Source: CAD feature listing. Evaluate the final solid. Frame: model axes, mm. Face numbers are marked on the shaded views. A direction names the side the tool comes from. Round coordinates to 2 decimals unless told otherwise and drop trailing zeros. Loops run counter-clockwise (first coordinate to the right, second up) from the corner with the lowest first, then second, coordinate; pieces in that order, holes last. Notation, with made-up numbers: (-21, 30) - (-2, 30) arc R22 ccw to (-2, 38) - close; hole circle Ø2 at (-28.5, -8). An arc over 180 degrees is marked (long way). One line per question, with ' | ' between items.
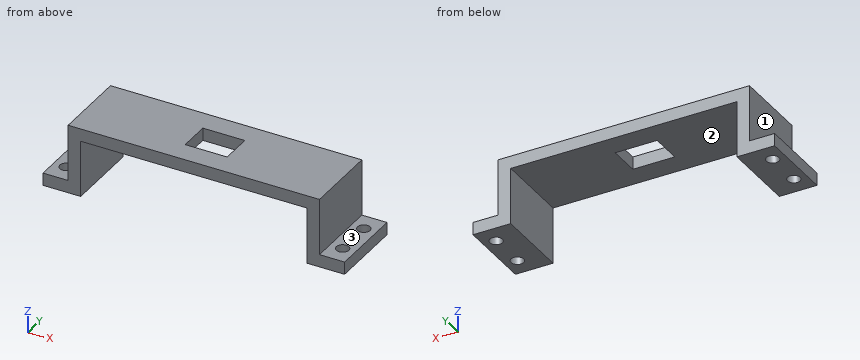
from build123d import *

# Parameters (mm, degrees)
SKETCH1_W           = 127
SKETCH1_H           = 38.1
SKETCH1_W_2         = 21.209
SKETCH1_H_2         = 15.88008
BOSS_EXTRUDE1_DEPTH = 6.35
SKETCH2_W           = 6.35
SKETCH2_H           = 38.1
BOSS_EXTRUDE2_DEPTH = 28.575
SKETCH3_W           = 6.35
SKETCH3_H           = 38.1
BOSS_EXTRUDE3_DEPTH = 12.7
SKETCH4_W           = 6.35
SKETCH4_H           = 38.1
BOSS_EXTRUDE4_DEPTH = 12.7
CUT_EXTRUDE1_REACH  = 149.595
SKETCH5_R           = 3.175


with BuildPart() as part:
    # Sketch1 → Boss-Extrude1 (new body)
    with BuildSketch(Plane.XY):
        with Locations((63.5, 19.05)):
            Rectangle(SKETCH1_W, SKETCH1_H)
        with Locations((63.5, 19.05)):
            Rectangle(SKETCH1_W_2, SKETCH1_H_2, mode=Mode.SUBTRACT)
    extrude(amount=BOSS_EXTRUDE1_DEPTH)

    # Sketch2 → Boss-Extrude2 (add)
    with BuildSketch(Plane(origin=(0, 0, 0), x_dir=(-1, 0, 0), z_dir=(0, 0, -1))):
        with Locations((-3.175, 19.05)):
            Rectangle(SKETCH2_W, SKETCH2_H)
        with Locations((-123.825, 19.05)):
            Rectangle(SKETCH2_W, SKETCH2_H)
    extrude(amount=BOSS_EXTRUDE2_DEPTH)

    # Sketch3 → Boss-Extrude3 (add)
    with BuildSketch(Plane(origin=(127, 0, 0), x_dir=(0, 0, -1), z_dir=(1, 0, 0))):
        with Locations((25.4, 19.05)):
            Rectangle(SKETCH3_W, SKETCH3_H)
    extrude(amount=BOSS_EXTRUDE3_DEPTH)

    # Sketch4 → Boss-Extrude4 (add)
    with BuildSketch(Plane.ZY):
        with Locations((-25.4, 19.05)):
            Rectangle(SKETCH4_W, SKETCH4_H)
    extrude(amount=BOSS_EXTRUDE4_DEPTH)

    # Sketch5 → Cut-Extrude1 (cut, up to next)
    with BuildSketch(Plane.XY.offset(-22.225), mode=Mode.PRIVATE) as cut_extrude1_sk1:
        with Locations((133.35, 28.575)):
            Circle(SKETCH5_R)
    cut_extrude1_tool1 = extrude(cut_extrude1_sk1.sketch, amount=-CUT_EXTRUDE1_REACH, mode=Mode.PRIVATE) & part.part
    # Sketch5 → Cut-Extrude1 (cut, up to next)
    with BuildSketch(Plane.XY.offset(-22.225), mode=Mode.PRIVATE) as cut_extrude1_sk2:
        with Locations((133.35, 9.525)):
            Circle(SKETCH5_R)
    cut_extrude1_tool2 = extrude(cut_extrude1_sk2.sketch, amount=-CUT_EXTRUDE1_REACH, mode=Mode.PRIVATE) & part.part
    # Sketch5 → Cut-Extrude1 (cut, up to next)
    with BuildSketch(Plane.XY.offset(-22.225), mode=Mode.PRIVATE) as cut_extrude1_sk3:
        with Locations((-6.35, 28.575)):
            Circle(SKETCH5_R)
    cut_extrude1_tool3 = extrude(cut_extrude1_sk3.sketch, amount=-CUT_EXTRUDE1_REACH, mode=Mode.PRIVATE) & part.part
    # Sketch5 → Cut-Extrude1 (cut, up to next)
    with BuildSketch(Plane.XY.offset(-22.225), mode=Mode.PRIVATE) as cut_extrude1_sk4:
        with Locations((-6.35, 9.525)):
            Circle(SKETCH5_R)
    cut_extrude1_tool4 = extrude(cut_extrude1_sk4.sketch, amount=-CUT_EXTRUDE1_REACH, mode=Mode.PRIVATE) & part.part
    add(cut_extrude1_tool1.solids().sort_by_distance((133.35, 28.575, -22.225))[0], mode=Mode.SUBTRACT)
    add(cut_extrude1_tool2.solids().sort_by_distance((133.35, 9.525, -22.225))[0], mode=Mode.SUBTRACT)
    add(cut_extrude1_tool3.solids().sort_by_distance((-6.35, 28.575, -22.225))[0], mode=Mode.SUBTRACT)
    add(cut_extrude1_tool4.solids().sort_by_distance((-6.35, 9.525, -22.225))[0], mode=Mode.SUBTRACT)


solid = part.part
1. Section query A-A, the plane x = -6.35. Return loops of the section in (y, z) (3 decimals).
Worked out:
outline: (0, -28.575) - (6.35, -28.575) - (6.35, -22.225) - (0, -22.225) - close; (12.7, -28.575) - (25.4, -28.575) - (25.4, -22.225) - (12.7, -22.225) - close; (31.75, -28.575) - (38.1, -28.575) - (38.1, -22.225) - (31.75, -22.225) - close
2. Access query for the marked faces 1, 2 and 3. Directions: +Z, -Z, +X, -X, +Y, -Y. A direction counts if a zero-diameter tool reaches every point of the face in a straight line with its end or side. Return the directions, or none.
Worked out:
face 1: +Z, -X, +Y, -Y | face 2: -Z, +Y, -Y | face 3: +Z, +X, +Y, -Y
3. Contact query for flat-ended pins moving along their axis: P1, Ø1.9, axis at y = 17.5, z = 3, coming from the -X side; P2, Ø5, axis at x = 133.35, y = 28.575, coming from the -Z side; P3, Ø1.9, axis at y = 21, z = 3.5, coming from the +X side; P4, Ø4, axis at x = 131, y = 13, coming from the +Z side (3 decimals). Output: stop coordinate, or through.
Worked out:
P1: stops at x = 0 | P2: passes through | P3: stops at x = 127 | P4: stops at z = -22.225
4. Material intervals for probe 1 along Y at (x, z) = (133, -24); probe 2 along X at (y, z) = (14.5, -14); probe 3 along X at (y, z) = (13, 4), sorted ascending.
Worked out:
probe 1: y = 0 to 6.37, 12.68 to 25.42, 31.73 to 38.1 | probe 2: x = 0 to 6.35, 120.65 to 127 | probe 3: x = 0 to 52.9, 74.1 to 127
5. Section query D-D, the plane y = 30. Return loops of the section in (x, z) (3 decimals).
Worked out:
outline: (-12.7, -28.575) - (-9.187, -28.575) - (-9.187, -22.225) - (-12.7, -22.225) - close; (-3.513, -28.575) - (6.35, -28.575) - (6.35, 0) - (120.65, 0) - (120.65, -28.575) - (130.513, -28.575) - (130.513, -22.225) - (127, -22.225) - (127, 6.35) - (0, 6.35) - (0, -22.225) - (-3.513, -22.225) - close; (136.187, -28.575) - (139.7, -28.575) - (139.7, -22.225) - (136.187, -22.225) - close
6. Section query B-B, the plane z = -26. Return loops of the section in (x, y) (3 decimals).
Worked out:
outline: (-12.7, 0) - (6.35, 0) - (6.35, 38.1) - (-12.7, 38.1) - close; (120.65, 0) - (139.7, 0) - (139.7, 38.1) - (120.65, 38.1) - close; hole circle Ø6.35 at (-6.35, 9.525); hole circle Ø6.35 at (-6.35, 28.575); hole circle Ø6.35 at (133.35, 9.525); hole circle Ø6.35 at (133.35, 28.575)
7. Section query C-C, the plane z = -10. Return loops of the section in (x, y).
Worked out:
outline: (0, 0) - (6.35, 0) - (6.35, 38.1) - (0, 38.1) - close; (120.65, 0) - (127, 0) - (127, 38.1) - (120.65, 38.1) - close
